Design review of the part built by this model. Coordinates are the model's own, in mm. A direction names the side the tool comes from. Coordinates: 2 decimals unless noted, no trailing zeros. Loops run counter-clockwise (first coordinate to the right, second up) from the corner with the lowest first, then second, coordinate; pieces in that order, holes last.
Q1. For P1, Ø8, axis at x = 17.5, z = 14.5, coming from the -Y side; P2, Ø2, axis at x = 17, y = -21.5, coming from the -Z side, all flat-tipped, find the tip position at first contact; note any pin that passes through.
Q2. Wall thickness on probe 1 along Y at (x, z) = (10, 17.25); probe 2 along X at (y, z) = (8, 5): over which ranges is each line inside the solid? List them lowest first.
Q3. Add section C-C on y = -50. Give the boundary of the cut face in (x, z).
Q4. Add section D-D on x = 5. Give the boundary of the cut face in (y, z).
Q5. Add section A-A on y = 15. Give the boundary of the cut face in (x, z).
Q6. Machinability: for faces 1 (the face through (10, 20, 12)), 2 (the face through (10, -30, 20)), 3 (the face through (16, -30, 22)), which of the approach directions +Z, -Z, +X, -X, +Y, -Y give a long, thin tool a straight path to every point of the face, cutting with its end or side? Answer none if there is none.
Q7. Draft analysis for pull direction X (two halves, no side actions). For faces 4 (the face through (10, 0, 10)), 5 (the face through (15, -7.5, 22)), 6 (the face through (0, 1, 13)), 7 (the face through (13.36, 12.77, 11.91)), state which applies: released by +X, released by -X, zero draft, split by the parting line, or undercut.
Q8. Add section B-B on x = 10. Give the boundary of the cut face in (y, z).
```python
from build123d import *

# Parameters (mm, degrees)
F0_W     = 20
F0_H     = 20
F1_DEPTH = 20
F2_W     = 20
F2_H     = 3.5
F3_DEPTH = 80
F4_R     = 2.75
F4_W     = 2
F4_H     = 5
F5_DEPTH = 3.5
F6_R     = 1.75
F6_R_2   = 0.9
F7_DEPTH = 23.5


with BuildPart() as f1:
    # F0 (on Top) → F1 (new body)
    with BuildSketch(Plane.XY):
        with Locations((10, 10)):
            Rectangle(F0_W, F0_H)
    extrude(amount=F1_DEPTH)

    # F2 (on face) → F3 (join)
    with BuildSketch(Plane(origin=(0, 20, 0), x_dir=(-1, 0, 0), z_dir=(0, 1, 0))):
        with Locations((-10, 21.75)):
            Rectangle(F2_W, F2_H)
    extrude(amount=-F3_DEPTH)

    # F4 (on face) → F5 (cut, through all)
    with BuildSketch(Plane.XY.offset(23.5)):
        with Locations((10, -50)):
            Circle(F4_R)
        with Locations((5, -10)):
            Rectangle(F4_W, F4_H)
        with Locations((5, -30)):
            Rectangle(F4_W, F4_H)
        with Locations((15, -10)):
            Rectangle(F4_W, F4_H)
        with Locations((15, -30)):
            Rectangle(F4_W, F4_H)
    extrude(amount=-F5_DEPTH, mode=Mode.SUBTRACT)

    # F6 (on face) → F7 (cut, through all)
    with BuildSketch(Plane.XY.offset(23.5)):
        with Locations((5, 15)):
            Circle(F6_R)
        with Locations((10, 15)):
            Circle(F6_R)
        with Locations((15, 15)):
            Circle(F6_R)
        with Locations((5, 10)):
            Circle(F6_R)
        with Locations((10, 10)):
            Circle(F6_R)
        with Locations((15, 10)):
            Circle(F6_R)
        with Locations((5, 5)):
            Circle(F6_R)
        with Locations((10, 5)):
            Circle(F6_R)
        with Locations((15, 5)):
            Circle(F6_R)
        with Locations((7.5, 12.5)):
            Circle(F6_R_2)
        with Locations((7.5, 7.5)):
            Circle(F6_R_2)
        with Locations((12.5, 12.5)):
            Circle(F6_R_2)
        with Locations((12.5, 7.5)):
            Circle(F6_R_2)
    extrude(amount=-F7_DEPTH, mode=Mode.SUBTRACT)


solid = f1.part
```
Entries:
1. P1: stops at y = 0
1. P2: stops at z = 20
2. probe 1: y = 0 to 3.25, 6.75 to 8.25, 11.75 to 13.25, 16.75 to 20
2. probe 2: x = 0 to 6.75, 8.25 to 11.75, 13.25 to 20
3. outline: (0, 20) - (7.25, 20) - (7.25, 23.5) - (0, 23.5) - close; (12.75, 20) - (20, 20) - (20, 23.5) - (12.75, 23.5) - close
4. outline: (-60, 20) - (-32.5, 20) - (-32.5, 23.5) - (-60, 23.5) - close; (-27.5, 20) - (-12.5, 20) - (-12.5, 23.5) - (-27.5, 23.5) - close; (-7.5, 20) - (0, 20) - (0, 0) - (3.25, 0) - (3.25, 23.5) - (-7.5, 23.5) - close; (6.75, 0) - (8.25, 0) - (8.25, 23.5) - (6.75, 23.5) - close; (11.75, 0) - (13.25, 0) - (13.25, 23.5) - (11.75, 23.5) - close; (16.75, 0) - (20, 0) - (20, 23.5) - (16.75, 23.5) - close
5. outline: (0, 0) - (3.25, 0) - (3.25, 23.5) - (0, 23.5) - close; (6.75, 0) - (8.25, 0) - (8.25, 23.5) - (6.75, 23.5) - close; (11.75, 0) - (13.25, 0) - (13.25, 23.5) - (11.75, 23.5) - close; (16.75, 0) - (20, 0) - (20, 23.5) - (16.75, 23.5) - close
6. face 1: +Z, -Z, +X, -X, +Y
6. face 2: -Z, +X, -X, -Y
6. face 3: +Z, -Z
7. face 4: zero draft
7. face 5: undercut
7. face 6: released by -X
7. face 7: undercut
8. outline: (-60, 20) - (-52.75, 20) - (-52.75, 23.5) - (-60, 23.5) - close; (-47.25, 20) - (0, 20) - (0, 0) - (3.25, 0) - (3.25, 23.5) - (-47.25, 23.5) - close; (6.75, 0) - (8.25, 0) - (8.25, 23.5) - (6.75, 23.5) - close; (11.75, 0) - (13.25, 0) - (13.25, 23.5) - (11.75, 23.5) - close; (16.75, 0) - (20, 0) - (20, 23.5) - (16.75, 23.5) - close
